The listing builds one solid part. Answer for the finished solid, in the listing's coordinates (mm). Coordinates: 2 decimals unless noted, no trailing zeros. Loops run counter-clockwise (first coordinate to the right, second up) from the corner with the lowest first, then second, coordinate; pieces in that order, holes last. Notation, with made-up numbers: (89, 44.25) - (135, 44.25) arc R18 ccw to (135, 60.25) - close; hole circle Ø8 at (21, 45). An arc over 180 degrees is marked (long way). Use one line per item in the form item = value. Start each with the question number.
```python
from build123d import *

# Parameters (mm, degrees)
SKETCH1_W               = 409
SKETCH1_H               = 122.5
BOSS_EXTRUDE1_DEPTH     = 2
CUT_EXTRUDE2_DEPTH      = 427.955793965
CUT_EXTRUDE2_DEPTH_BACK = 427.955793965
SKETCH2_W               = 17
SKETCH2_H               = 8.53
SKETCH2_W_2             = 10
SKETCH2_H_2             = 7.25


with BuildPart() as part:
    # Sketch1 → Boss-Extrude1 (new body)
    with BuildSketch(Plane.XY):
        with Locations((204.5, -61.25)):
            Rectangle(SKETCH1_W, SKETCH1_H)
    extrude(amount=BOSS_EXTRUDE1_DEPTH)

    # Sketch2 → Cut-Extrude2 (cut, two sides: drawn at the far end of the back side and taken through both)
    with BuildSketch(Plane.XY.offset(2).offset(-CUT_EXTRUDE2_DEPTH_BACK)):
        with Locations((12.9, -17.865)):
            Rectangle(SKETCH2_W, SKETCH2_H)
        with Locations((51, -17.865)):
            Rectangle(SKETCH2_W, SKETCH2_H)
        with Locations((89.1, -17.865)):
            Rectangle(SKETCH2_W, SKETCH2_H)
        with Locations((127.2, -17.865)):
            Rectangle(SKETCH2_W, SKETCH2_H)
        with Locations((165.3, -17.865)):
            Rectangle(SKETCH2_W, SKETCH2_H)
        with Locations((203.4, -17.865)):
            Rectangle(SKETCH2_W, SKETCH2_H)
        with Locations((279.6, -17.865)):
            Rectangle(SKETCH2_W, SKETCH2_H)
        with Locations((241.5, -17.865)):
            Rectangle(SKETCH2_W, SKETCH2_H)
        with Locations((317.7, -17.865)):
            Rectangle(SKETCH2_W, SKETCH2_H)
        with Locations((348.775, -17.225)):
            Rectangle(SKETCH2_W_2, SKETCH2_H_2)
        with BuildLine():
            Line((280.1, -85.45), (280.1, -83.595607239))
            ThreePointArc((280.1, -83.595607239), (279, -61.35), (277.9, -83.595607239))
            Line((277.9, -83.595607239), (277.9, -85.45))
            Line((277.9, -85.45), (280.1, -85.45))
        make_face()
    extrude(amount=CUT_EXTRUDE2_DEPTH + CUT_EXTRUDE2_DEPTH_BACK, mode=Mode.SUBTRACT)


solid = part.part
```
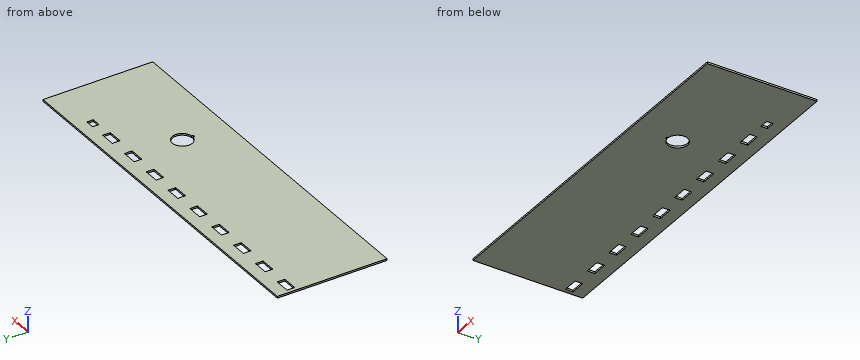
(1) A cutting plane is placed at A-A (y = -72.5). Determine the outline of the cut face in (x, z).
(2) Find the intervals of material crossed by probe 1 along Y at (x, z) = (279, 1.25); probe 2 along X at (y, z) = (-72.5, 1.6); probe 3 along Y at (x, z) = (122.5, 0.8), in increasing order. Write a range as from..to.
(3) A cutting plane is placed at C-C (z = 1.6). State how many separate pieces and enclosed holes the cut face has, then the cut area to 3 significant figures.
(4) A cutting plane is placed at B-B (x = 203). Determine the outline of the cut face in (y, z), then the cut area to 3 significant figures.
Evaluation:
q1.outline = (0, 0) - (267.85, 0) - (267.85, 2) - (0, 2) - close; (290.15, 0) - (409, 0) - (409, 2) - (290.15, 2) - close
q2.probe_1 = -122.5..-85.45, -61.35..-22.13, -13.6..0
q2.probe_2 = 0..267.85, 290.15..409
q2.probe_3 = -122.5..-22.13, -13.6..0
q3.separate_pieces = 1
q3.enclosed_holes = 11
q3.area = 48,300 mm^2
q4.outline = (-122.5, 0) - (-22.13, 0) - (-22.13, 2) - (-122.5, 2) - close; (-13.6, 0) - (0, 0) - (0, 2) - (-13.6, 2) - close
q4.area = 228 mm^2
